Autodesk Inventor part; units mm, degrees
ref_plane "YZ Plane" through (0, 0, 0) normal (1, 0, 0) x (0, 1, 0)
ref_plane "XZ Plane" through (0, 0, 0) normal (0, 1, 0) x (-1, 0, 0)
ref_plane "XY Plane" through (0, 0, 0) normal (0, 0, 1) x (1, 0, 0)
sketch "Sketch1" plane through (0, 0, 0) normal (0, 0, 1) x (1, 0, 0)
  line L0 (-47.5, 35) -> (47.5, 35)
  line L1 (47.5, 35) -> (47.5, -35)
  line L2 (47.5, -35) -> (-47.5, -35)
  line L3 (-47.5, -35) -> (-47.5, 35)
  point P0 (0, 0)
  point P1 (0, 35)
  point P2 (-47.5, 0)
  dimension "d0" = 95
  dimension "d1" = 70
extrude "Extrusion1" add sketch "Sketch1" along normal blind 10
sketch "Sketch2" plane through (0, 0, 0) normal (0, 0, -1) x (-1, 0, 0)
  line L0 (0, 71.7114) -> (0, -41.7697) construction
  line L1 (-47.5, 35) -> (47.5, 35) construction
  line L2 (-22.5, 19.157) -> (-23.5, 19.157)
  circle A0 centre (35, -20) radius 8.5
  line L3 (47.5, -35) -> (-47.5, -35)
  line L4 (-47.5, -35) -> (-47.5, 35)
  circle A1 centre (43.4853, -28.4853) radius 2.25
  line L5 (47.5, 35) -> (47.5, -35) construction
  line L6 (26.5147, -11.5147) -> (43.4853, -11.5147) construction
  line L7 (43.4853, -11.5147) -> (43.4853, -28.4853) construction
  line L8 (43.4853, -28.4853) -> (26.5147, -28.4853) construction
  line L9 (26.5147, -28.4853) -> (26.5147, -11.5147) construction
  circle A2 centre (43.4853, -11.5147) radius 2.25
  circle A3 centre (26.5147, -11.5147) radius 2.25
  circle A4 centre (26.5147, -28.4853) radius 2.25
  circle A5 centre (-35, -20) radius 8.5
  circle A6 centre (-43.4853, -28.4853) radius 2.25
  circle A7 centre (-43.4853, -11.5147) radius 2.25
  circle A8 centre (-26.5147, -11.5147) radius 2.25
  circle A9 centre (-26.5147, -28.4853) radius 2.25
  point P0 (0, 0)
  point P1 (0, 14.9709)
  point P2 (0, 35)
  point P3 (35, -11.5147)
  point P4 (26.5147, -20)
  dimension "d21" = 15
  dimension "d22" = 12.5
  dimension "d23" = 17
  dimension "d26" = 4.5
  dimension "d27" = 16.9706
  dimension "d28" = 16.9706
extrude "Extrusion2" cut sketch "Sketch2" against normal through all
sketch "Sketch3" plane through (0, 0, 0) normal (0, 0, -1) x (-1, 0, 0)
  circle A0 centre (0, -3.4021) radius 5.75
  circle A1 centre (35, -20) radius 8.5
  line L0 (-47.5, 35) -> (47.5, 35)
  line L1 (47.5, 35) -> (47.5, -35)
  line L2 (47.5, -35) -> (-47.5, -35)
  line L3 (-47.5, -35) -> (-47.5, 35)
  circle A2 centre (35, -20) radius 8.5
  circle A3 centre (0, 4.5979) radius 2
  circle A4 centre (-8, -3.4021) radius 2
  circle A5 centre (0, -11.4021) radius 2
  circle A6 centre (8, -3.4021) radius 2
  circle A7 centre (26.5147, -11.5147) radius 2.25
  circle A8 centre (-43.4853, -28.4853) radius 2.25
  circle A9 centre (-43.4853, -11.5147) radius 2.25
  circle A10 centre (26.5147, -28.4853) radius 2.25
  circle A11 centre (43.4853, -11.5147) radius 2.25
  circle A12 centre (-26.5147, -28.4853) radius 2.25
  circle A13 centre (-26.5147, -11.5147) radius 2.25
  circle A14 centre (43.4853, -28.4853) radius 2.25
  circle A15 centre (26.5147, -11.5147) radius 2.25
  circle A16 centre (-43.4853, -28.4853) radius 2.25
  circle A17 centre (-43.4853, -11.5147) radius 2.25
  circle A18 centre (26.5147, -28.4853) radius 2.25
  circle A19 centre (43.4853, -11.5147) radius 2.25
  circle A20 centre (-26.5147, -28.4853) radius 2.25
  circle A21 centre (-26.5147, -11.5147) radius 2.25
  circle A22 centre (43.4853, -28.4853) radius 2.25
  circle A23 centre (-35, -20) radius 8.5
  circle A24 centre (-35, -20) radius 8.5
  line L4 (-47.5, 35) -> (47.5, 35)
  line L5 (47.5, 35) -> (47.5, -35)
  line L6 (47.5, -35) -> (-47.5, -35)
  line L7 (-47.5, -35) -> (-47.5, 35)
  point P0 (0, 0)
  point P1 (1.1874, 2.9885)
  point P2 (-1.1874, 2.9885)
  point P3 (0, -3.4021)
  point P4 (0, -35)
  dimension "d10" = 31.5979
  dimension "d12" = 11.5
  dimension "d13" = 4
  dimension "d14" = 8
  dimension "d19" = 360
extrude "Extrusion3" cut sketch "Sketch3" against normal through all contours A0 | A3 | A4 | A5 | A6
sketch "Sketch5" plane through (0, 0, 0) normal (0, 0, -1) x (-1, 0, 0)
  circle A0 centre (19.75, 31) radius 2
  circle A1 centre (19.75, 12) radius 2
  line L0 (47.5, 35) -> (47.5, -35)
  line L1 (-47.5, 35) -> (47.5, 35)
  point P0 (0, 0)
  dimension "d29" = 27.75
  dimension "d30" = 4
  dimension "d31" = 4
  dimension "d32" = 19
hole "Hole1" at (-19.75, 12, 0) at (-19.75, 31, 0) direction (0, 0, 1) diameter 4 depth 11 tip angle 118 counterbore diameter 7 counterbore depth 3
sketch "Sketch6" plane through (0, 0, 0) normal (0, 0, -1) x (-1, 0, 0)
  line L0 (23.25, 27.5) -> (16.25, 27.5)
  line L1 (16.25, 27.5) -> (16.25, 35)
  line L2 (16.25, 35) -> (23.25, 35)
  line L3 (23.25, 35) -> (23.25, 27.5)
  line L4 (-47.5, 35) -> (47.5, 35)
  circle A0 centre (19.75, 31) radius 3.5
  point P0 (0, 0)
  point P1 (16.25, 31)
  point P2 (23.25, 31)
extrude "Extrusion4" cut sketch "Sketch6" against normal up to surface (3 mm away) contours A0 L1 L2 L3
mirror "Mirror1" about plane through (0, 0, 0) normal (1, 0, 0) of "Extrusion4", "Hole1"
chamfer "Chamfer1" distance 7 angle 45 2 edges at (-47.5, 35, 5) (47.5, 35, 5)
equation "\"BendRadius\" = Thickness"
equation "\"BendReliefWidth\" = Thickness"
equation "\"BendReliefDepth\" = 0.5 * Thickness"
equation "\"CornerReliefSize\" = 4 * Thickness"
equation "\"MinimumRemnant\" = 2 * Thickness"
equation "\"TransitionRadius\" = BendRadius"
equation "\"JacobiRadiusSize\" = Thickness"
equation "\"GapSize\" = Thickness"
properties part number "0008-10-001" material "ABS Plastic"
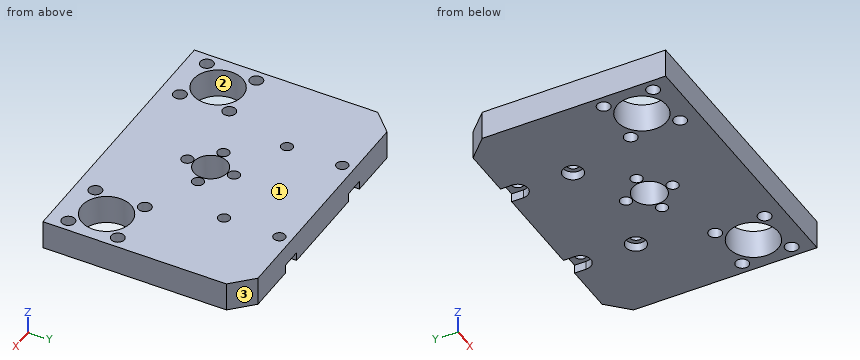
Model file for the job. Use its own axes, mm. Face numbers are marked on the shaded views. Give positions to 0.01 mm unless a question says otherwise; leave off trailing zeros. Order: outer loops, then holes, each group sorted by start corner. A loop starts at its lowest first (then second) coordinate and runs counter-clockwise, first axis right, second up. Notation, with made-up numbers: (40, 2) - (62, 2) arc R18 cw to (62, 31) - close; hole circle Ø1 at (-30, 7.5). An arc over 180 degrees is marked (long way). Write item = value, one per line. Start each with the question number.
1. Drop flat-ended pins along their axis: P1, Ø3.5, axis at y = 32.5, z = 2, coming from the -X side; P2, Ø3.5, axis at x = -20, y = 11, coming from the -Z side. Give the stop position or say it passes through.
2. Cut at A-A, the plane y = 12. List the corners of the cut face in (x, z).
3. Cut at D-D, the plane z = 7.25. State how many separate pieces and enclosed holes the cut face has, and give its area (3 significant figures).
4. Probe line 1 along Y through (x, z) = (-19.75, 7.5); line 2 along Y through (x, z) = (35, 3); line 3 along Y through (x, z) = (0, 7). List the from-to ranges inside material, lowest first.
5. Cut at C-C, the plane x = -35. List the corners of the cut face in (y, z), and give its area (3 significant figures).
6. Two-plate mould, pull along X, no slides. Class the marked faces 1, 2 and 3: pulls with the +X half, pulls with the -X half, needs draft (parallel to the pull), parting line crosses it, or undercut.
7. Cut at B-B, the plane x = 19.75. List the corners of the cut face in (y, z), and give its area (4 significant figures).
Taken from the geometry:
q1.P1 = -44.75
q1.P2 = 3
q2.outline = (-47.5, 0) - (-23.25, 0) - (-23.25, 3) - (-21.75, 3) - (-21.75, 10) - (-47.5, 10) - close; (-17.75, 3) - (-16.25, 3) - (-16.25, 0) - (16.25, 0) - (16.25, 3) - (17.75, 3) - (17.75, 10) - (-17.75, 10) - close; (21.75, 3) - (23.25, 3) - (23.25, 0) - (47.5, 0) - (47.5, 10) - (21.75, 10) - close
q3.separate_pieces = 1
q3.enclosed_holes = 19
q3.area = 5,820 mm²
q4.line_1 = -35 to 10, 14 to 29, 33 to 35
q4.line_2 = -35 to -28.5, -11.5 to 35
q4.line_3 = -35 to -13.4, -9.4 to -9.15, 2.35 to 2.6, 6.6 to 35
q5.outline = (-35, 0) - (-28.5, 0) - (-28.5, 10) - (-35, 10) - close; (-11.5, 0) - (35, 0) - (35, 10) - (-11.5, 10) - close
q5.area = 530 mm²
q6.face_1 = needs draft
q6.face_2 = undercut
q6.face_3 = pulls with the +X half
q7.outline = (-35, 0) - (8.5, 0) - (8.5, 3) - (10, 3) - (10, 10) - (-35, 10) - close; (14, 3) - (15.5, 3) - (15.5, 0) - (27.5, 0) - (27.5, 3) - (29, 3) - (29, 10) - (14, 10) - close; (33, 3) - (35, 3) - (35, 10) - (33, 10) - close
q7.area = 600.5 mm²
